Source: CAD feature listing. Evaluate the final solid. Frame: model axes, mm. Give positions to 0.01 mm unless a question says otherwise; leave off trailing zeros. Loops run counter-clockwise (first coordinate to the right, second up) from the corner with the lowest first, then second, coordinate; pieces in that order, holes last. Notation, with made-up numbers: (-29.75, 35.25) -> (20.25, 35.25) arc R17 cw to (20.25, 59.25) -> close; hole circle Ø9 at (61.5, -11.5). An arc over 180 degrees is marked (long way). Put each result on its own line as item: value.
```python
from build123d import *

# Parameters (mm, degrees)
CYLINDER053_R          = 2
CYLINDER053_DEPTH      = 10
CYLINDER054_R          = 2
CYLINDER054_DEPTH      = 10
BOX014_W               = 14
BOX014_H               = 3
BOX014_DEPTH           = 20
BOX014_PLACEMENT_ANGLE = -90
CHAMFER015_SIZE        = 1
CHAMFER017_SIZE        = 1


with BuildPart() as cilindro050:
    # Cylinder053 → Cylinder053 (new body)
    with BuildSketch(Plane(origin=(63, -53, 25), x_dir=(0, -1, 0), z_dir=(-1, 0, 0))):
        Circle(CYLINDER053_R)
    extrude(amount=CYLINDER053_DEPTH)


with BuildPart() as fusion013:
    # Cylinder054 → Cylinder054 (new body)
    with BuildSketch(Plane(origin=(63, -53, 37), x_dir=(0, -1, 0), z_dir=(-1, 0, 0))):
        Circle(CYLINDER054_R)
    extrude(amount=CYLINDER054_DEPTH)

    # Fusion013: union Cilindro050
    add(cilindro050.part)


with BuildPart() as obj1:
    # Box014 → Box014 (new body)
    with BuildSketch(Plane.XY):
        with Locations((7, 1.5)):
            Rectangle(BOX014_W, BOX014_H)
    extrude(amount=BOX014_DEPTH)


with BuildPart() as obj1_1:
    # Box014 placement: moved
    add(obj1.part.moved(Location((55, -48, 21))).rotate(Axis((55, -48, 21), (0, 0, 1)), BOX014_PLACEMENT_ANGLE))

    # Cut041: cut Fusion013
    add(fusion013.part, mode=Mode.SUBTRACT)


with BuildPart() as obj1_2:
    # Cut041 placement: moved
    add(obj1_1.part.moved(Location((-7, 0, 0))))

    # Chamfer015
    chamfer015_edges = [obj1_2.edges().sort_by_distance(p)[0] for p in [
        (49.5, -62, 41),
        (49.5, -62, 21),
    ]]
    chamfer(chamfer015_edges, length=CHAMFER015_SIZE)

    # Chamfer017
    chamfer017_edges = [obj1_2.edges().sort_by_distance(p)[0] for p in [
        (48, -48, 31),
        (48, -62, 31),
    ]]
    chamfer(chamfer017_edges, length=CHAMFER017_SIZE)


solid = obj1_2.part
```
(1) Line query: probe 1 along Z at (x, y) = (49.8, -53); probe 2 along Y at (x, z) = (49.6, 25); probe 3 along Z at (x, y) = (48.9, -54.75). Output: solid intervals per line, ascending. Write a range as from..to.
Calculated:
probe 1: z = 21..23, 27..35, 39..41
probe 2: y = -62..-55, -51..-48
probe 3: z = 21..24.03, 25.97..36.03, 37.97..41
(2) Draft query along Z for faces 1 (the flat face through (48, -55, 31)), 2 (the cylindrical face through (50, -53, 35)), 3 (the flat face through (49.8, -61.5, 40.5)). Return one class per face: released by +Z, released by -Z, zero draft, split by the parting line, or undercut.
Calculated:
face 1: zero draft
face 2: undercut
face 3: released by +Z
(3) Section A-A on x = 48.25. Return loops of the section in (y, z), then the cut area to 3 significant figures.
Calculated:
outline: (-61.25, 21.25) -> (-61, 21) -> (-48.75, 21) -> (-48.75, 41) -> (-61, 41) -> (-61.25, 40.75) -> close; hole circle Ø4 at (-53, 25); hole circle Ø4 at (-53, 37)
area: 225 mm²
(4) First-contact query: P1, Ø4.5, axis at y = -53, z = 37, coming from the -X side. Flat tip, straight axial feed; report the tip coordinate or a pass-through.
Calculated:
P1: stops at x = 48
(5) Section C-C on y = -53. Return loops of the section in (x, z), then the cut area to 3 significant figures.
Calculated:
outline: (48, 21) -> (51, 21) -> (51, 23) -> (48, 23) -> close; (48, 27) -> (51, 27) -> (51, 35) -> (48, 35) -> close; (48, 39) -> (51, 39) -> (51, 41) -> (48, 41) -> close
area: 36.0 mm²
(6) Section B-B on z = 37. Return loops of the section in (x, y).
Calculated:
outline: (48, -61) -> (49, -62) -> (51, -62) -> (51, -55) -> (48, -55) -> close; (48, -51) -> (51, -51) -> (51, -48) -> (49, -48) -> (48, -49) -> close
(7) Section D-D on z = 30.75. Return loops of the section in (x, y).
Calculated:
outline: (48, -61) -> (49, -62) -> (51, -62) -> (51, -48) -> (49, -48) -> (48, -49) -> close
